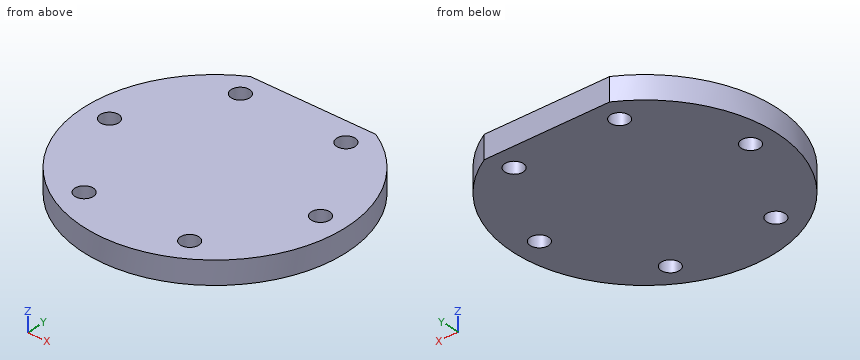
from build123d import *

# Parameters (mm, degrees)
SKETCH_1_R      = 2
EXTRUDE_1_DEPTH = 5


with BuildPart() as part:
    # 草图1 → 凸台-拉伸1 (new body)
    with BuildSketch(Plane.XY):
        with BuildLine():
            Line((-13.683932183, 25), (13.683932183, 25))
            ThreePointArc((13.683932183, 25), (0, -28.5), (-13.683932183, 25))
        make_face()
        with Locations((23, 0)):
            Circle(SKETCH_1_R, mode=Mode.SUBTRACT)
        with Locations((11.5, -19.918584287)):
            Circle(SKETCH_1_R, mode=Mode.SUBTRACT)
        with Locations((-11.5, -19.918584287)):
            Circle(SKETCH_1_R, mode=Mode.SUBTRACT)
        with Locations((-23, 0)):
            Circle(SKETCH_1_R, mode=Mode.SUBTRACT)
        with Locations((-11.5, 19.918584287)):
            Circle(SKETCH_1_R, mode=Mode.SUBTRACT)
        with Locations((11.5, 19.918584287)):
            Circle(SKETCH_1_R, mode=Mode.SUBTRACT)
    extrude(amount=EXTRUDE_1_DEPTH)


solid = part.part
Part model, mm, in its own coordinate system. Coordinates: 2 decimals unless noted, no trailing zeros. Loops run counter-clockwise (first coordinate to the right, second up) from the corner with the lowest first, then second, coordinate; pieces in that order, holes last. Notation, with made-up numbers: (7.5, -30.75) -> (30.5, -30.75) arc R9 ccw to (30.5, -23.75) -> close; hole circle Ø6 at (73, 2.5). An arc over 180 degrees is marked (long way). Use a Markdown table: item, result. Add a question column.
Item 1: Band-saw the part on A-A on y = 0. Write the cut outline in (x, z), plus the area to 3 significant figures.
Item 2: Band-saw the part on B-B on x = 23. Write the cut outline in (y, z).
Item 3: Probe probe 1 along Y at (x, z) = (10.5, 2.5); probe 2 along X at (y, z) = (21, 4.45); probe 3 along X at (y, z) = (-19, 3.75). List the from-to ranges inside material, lowest first.
Item 4: Band-saw the part on D-D on x = 11.5. Write the cut outline in (y, z).
Item 5: Flat gauge pins, fed straight in: P1, Ø1.5, axis at x = 9.5, z = 0.5, coming from the -Y side; P2, Ø1, axis at x = -19, y = 16.5, coming from the -Z side. Where does each tip first touch, or does it go through?
Item 6: Band-saw the part on C-C on z = 3.8. Write the cut outline in (x, y), plus the area to 3 significant figures.
Geometry says:
| question | item | result |
|---|---|---|
| 1 | outline | (-28.5, 0) -> (-25, 0) -> (-25, 5) -> (-28.5, 5) -> close; (-21, 0) -> (21, 0) -> (21, 5) -> (-21, 5) -> close; (25, 0) -> (28.5, 0) -> (28.5, 5) -> (25, 5) -> close |
| 1 | area | 245 mm² |
| 2 | outline | (-16.83, 0) -> (-2, 0) -> (-2, 5) -> (-16.83, 5) -> close; (2, 0) -> (16.83, 0) -> (16.83, 5) -> (2, 5) -> close |
| 3 | probe 1 | -26.5 to -21.65, -18.19 to 18.19, 21.65 to 25 |
| 3 | probe 2 | -19.27 to -13.18, -9.82 to 9.82, 13.18 to 19.27 |
| 3 | probe 3 | -21.24 to -13.28, -9.72 to 9.72, 13.28 to 21.24 |
| 4 | outline | (-26.08, 0) -> (-21.92, 0) -> (-21.92, 5) -> (-26.08, 5) -> close; (-17.92, 0) -> (17.92, 0) -> (17.92, 5) -> (-17.92, 5) -> close; (21.92, 0) -> (25, 0) -> (25, 5) -> (21.92, 5) -> close |
| 5 | P1 | y = -27.12 |
| 5 | P2 | z = 0 |
| 6 | outline | (-13.68, 25) arc R28.5 ccw (long way) to (13.68, 25) -> close; hole circle Ø4 at (-23, 0); hole circle Ø4 at (-11.5, -19.92); hole circle Ø4 at (-11.5, 19.92); hole circle Ø4 at (11.5, -19.92); hole circle Ø4 at (11.5, 19.92); hole circle Ø4 at (23, 0) |
| 6 | area | 2,410 mm² |
